```python
from build123d import *

# Parameters (mm, degrees)
F1_DEPTH = 11.5
F2_R     = 1.2
F3_DEPTH = 25
F4_R     = 2.5
F5_W     = 12
F5_H     = 9.5
F6_DEPTH = 10.001
F7_W     = 6
F7_H     = 3
F8_DEPTH = 13.001


with BuildPart() as f1:
    # F0 (on Top) → F1 (new body)
    with BuildSketch(Plane.XY):
        Polygon((-13.5, 5.5), (-13.5, 0), (-6, 0), (-6, 10), (6, 10), (6, 0), (13.5, 0), (13.5, 5.5), (9, 13), (-9, 13), align=None)
    extrude(amount=F1_DEPTH)

    # F2 (on face) → F3 (cut)
    with BuildSketch(Plane.XZ):
        with Locations((-9, 7.2)):
            Circle(F2_R)
        with Locations((9, 7.2)):
            Circle(F2_R)
    extrude(amount=-F3_DEPTH, mode=Mode.SUBTRACT)

    # F4
    f4_edges = [f1.edges().sort_by_distance(p)[0] for p in [
        (-6, 10, 5.75),
        (6, 10, 5.75),
    ]]
    fillet(f4_edges, radius=F4_R)

    # F5 (on face) → F6 (cut, through all)
    with BuildSketch(Plane.XZ.offset(-10)):
        with Locations((0, 6.75)):
            Rectangle(F5_W, F5_H)
    extrude(amount=F6_DEPTH, mode=Mode.SUBTRACT)

    # F7 (on face) → F8 (cut, through all)
    with BuildSketch(Plane.XZ):
        with Locations((-10.5, 1.5)):
            Rectangle(F7_W, F7_H)
        with Locations((10.5, 1.5)):
            Rectangle(F7_W, F7_H)
    extrude(amount=-F8_DEPTH, mode=Mode.SUBTRACT)


solid = f1.part
```
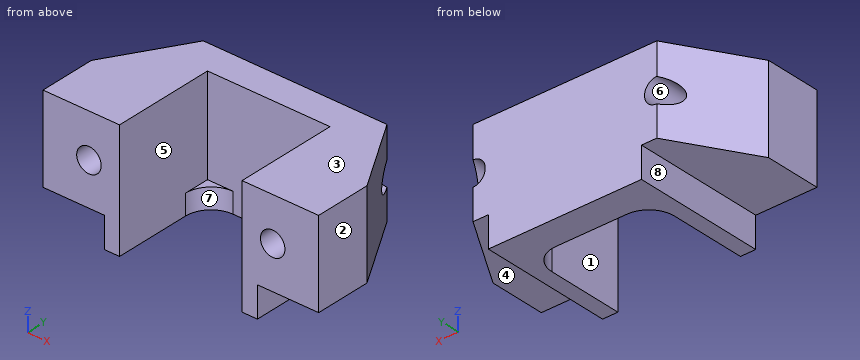
Source: CAD feature listing. Evaluate the final solid. Frame: model axes, mm. Face numbers are marked on the shaded views. A direction names the side the tool comes from. Round coordinates to 2 decimals unless told otherwise and drop trailing zeros. Loops run counter-clockwise (first coordinate to the right, second up) from the corner with the lowest first, then second, coordinate; pieces in that order, holes last. Notation, with made-up numbers: (-18.75, -25.75) - (16.25, -25.75) arc R18 ccw to (16.25, -17.75) - close; hole circle Ø1 at (-25.5, 78). An arc over 180 degrees is marked (long way). Use CSV: the item, a comma, the result in double quotes.
Q1. Section query C-C, the plane x = 9.5. Output: boundary loops of the cut face in (y, z).
Reported:
outline,"(0, 3) - (12.17, 3) - (12.17, 6.11) - (0, 6.11) - close; (0, 8.29) - (12.17, 8.29) - (12.17, 11.5) - (0, 11.5) - close"
Q2. Reachability of the marked faces 4, 5, 6, 7 and 8 from +Z, -Z, +X, -X, +Y, -Y: full face, straight path, thin tool, end or side. Return the list, or none.
Reported:
face 4,"-Z, +X, +Y, -Y"
face 5,"+Z, -Y"
face 6,"+Y, -Y"
face 7,"+Z, -Z, -Y"
face 8,"-Z, -X, +Y, -Y"
Q3. Mould query, pull axis X, two halves, no side actions, for the marked faces 1, 2 and 3. Classes: pulls with the +X half, pulls with the -X half, needs draft (parallel to the pull), parting line crosses it, or undercut.
Reported:
face 1,"undercut"
face 2,"pulls with the +X half"
face 3,"needs draft"
Q4. Section query B-B, the plane y = 3. Output: boundary loops of the cut face in (x, z).
Reported:
outline,"(-13.5, 3) - (-7.5, 3) - (-7.5, 0) - (-6, 0) - (-6, 11.5) - (-13.5, 11.5) - close; (6, 0) - (7.5, 0) - (7.5, 3) - (13.5, 3) - (13.5, 11.5) - (6, 11.5) - close; hole circle Ø2.4 at (-9, 7.2); hole circle Ø2.4 at (9, 7.2)"
Q5. Section query A-A, the plane z = 7.2. Output: boundary loops of the cut face in (x, y).
Reported:
outline,"(-13.5, 0) - (-10.2, 0) - (-10.2, 11) - (-13.5, 5.5) - close; (-7.8, 0) - (-6, 0) - (-6, 10) - (6, 10) - (6, 0) - (7.8, 0) - (7.8, 13) - (-7.8, 13) - close; (10.2, 0) - (13.5, 0) - (13.5, 5.5) - (10.2, 11) - close"
Q6. Ray query, line 1 along X through (y, z) = (3.75, 7.2); line 2 along Z through (x, y) = (-9, 7.75); line 3 along X through (y, z) = (7.25, 2). Return the intervals inside material, ascending.
Reported:
line 1,"-13.5 to -10.2, -7.8 to -6, 6 to 7.8, 10.2 to 13.5"
line 2,"3 to 6, 8.4 to 11.5"
line 3,"-7.5 to -6, 6 to 7.5"
Q7. Section query D-D, the plane z = 1.5. Output: boundary loops of the cut face in (x, y).
Reported:
outline,"(-7.5, 0) - (-6, 0) - (-6, 7.5) arc R2.5 cw to (-3.5, 10) - (3.5, 10) arc R2.5 cw to (6, 7.5) - (6, 0) - (7.5, 0) - (7.5, 13) - (-7.5, 13) - close"
Q8. Pin query (flat end, axial travel): pin 1 Ø6 at (x, z) = (3.5, 3) entering from -Y; pin 2 Ø2 at (y, z) = (11, 2.5) entering from -X; pin 3 Ø3 at (x, y) = (-10.5, 5.5) entering from -Z; pin 4 Ø6 at (y, z) = (9.5, 4) entering from -X. Return the tip coordinate at first contact, or that it passes through.
Reported:
pin 1,"y = 0"
pin 2,"x = -10.72"
pin 3,"z = 3"
pin 4,"x = -12.9"
